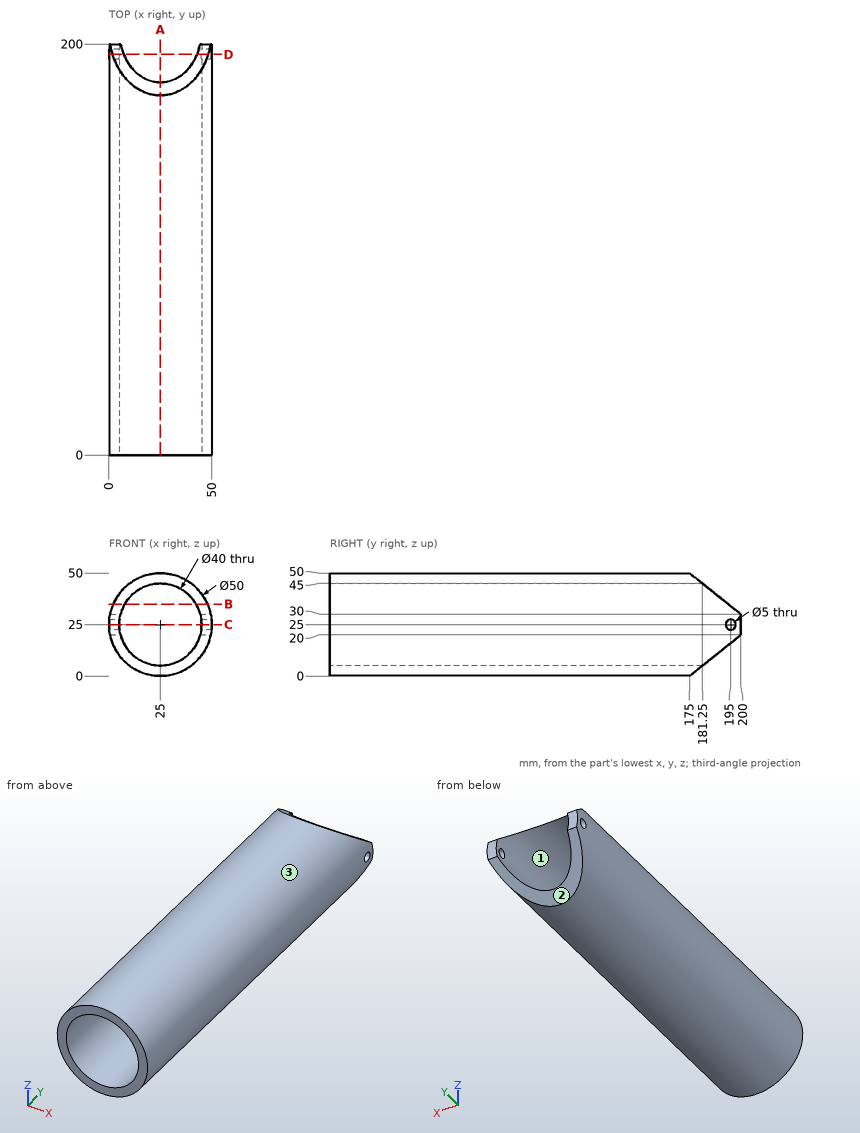
The drawing under review shows one solid part. Ordinate dimensions are in mm from its lowest x, y, z. Give positions to 0.01 mm unless a question says otherwise; leave off trailing zeros. Write each loop counter-clockwise with the first axis right and the second up, starting at its lowest first coordinate (ties: lowest second). Pieces come first, ordered by that corner, then holes.
1. Add section A-A, the plane x = 25. Write out the cut boundary in (y, z), plus the area to 3 significant figures.
2. For P1, Ø4, axis at x = 21, y = 164.5, coming from the +Z side; P2, Ø3, axis at y = 22, z = 36.5, coming from the -X side; P3, Ø4, axis at y = 24.5, z = 8, coming from the +X side, all flat-tipped, find the tip position at first contact; note any pin that passes through.
3. Draft analysis for pull direction X (two halves, no side actions). For the marked faces 1, 2 and 3, state which applies: +X half, -X half, draft (parallel to the pull), parting line (faces both ways), or undercut.
4. Add section C-C, the plane z = 25. Write out the cut boundary in (x, y), plus the area to 3 significant figures.
5. Wall thickness on L1, parallel to Y at x = 2.35, z = 25; L2, parallel to X at y = 15, z = 25; L3, parallel to X at y = 175, z = 17.5: over which ranges is each line inside the solid? List them lowest first.
6. Add section B-B, the plane z = 35. Write out the cut boundary in (x, y), plus the area to 3 significant figures.
7. Add section D-D, the plane y = 195. Write out the cut boundary in (x, z), plus the area to 3 significant figures.
Worked answers:
1. outline: (0, 0) - (175, 0) - (181.25, 5) - (0, 5) - close; (0, 45) - (181.25, 45) - (175, 50) - (0, 50) - close
1. area: 1,780 mm2
2. P1: stops at z = 49.92
2. P2: stops at x = 2.09
2. P3: stops at x = 45
3. face 1: undercut
3. face 2: draft
3. face 3: parting line
4. outline: (0, 0) - (5, 0) - (5, 192.5) - (0, 192.5) - close; (0, 197.5) - (5, 197.5) - (5, 200) - (0, 200) - close; (45, 0) - (50, 0) - (50, 192.5) - (45, 192.5) - close; (45, 197.5) - (50, 197.5) - (50, 200) - (45, 200) - close
4. area: 1,950 mm2
5. L1: y = 0 to 192.5, 197.5 to 200
5. L2: x = 0 to 5, 45 to 50
5. L3: x = 1.15 to 6.46, 43.54 to 48.85
6. outline: (2.09, 0) - (7.68, 0) - (7.68, 193.75) - (2.09, 193.75) - close; (42.32, 0) - (47.91, 0) - (47.91, 193.75) - (42.32, 193.75) - close
6. area: 2,170 mm2
7. outline: (0.13, 22.5) arc R25 ccw to (1.68, 16) - (7.14, 16) arc R20 cw to (5.16, 22.5) - close; (0.13, 27.5) - (5.16, 27.5) arc R20 cw to (7.14, 34) - (1.68, 34) arc R25 ccw to start; (42.86, 16) - (48.32, 16) arc R25 ccw to (49.87, 22.5) - (44.84, 22.5) arc R20 cw to start; (42.86, 34) arc R20 cw to (44.84, 27.5) - (49.87, 27.5) arc R25 ccw to (48.32, 34) - close
7. area: 135 mm2
